Could you check a few things on this model? Use its own coordinates, in mm. Face numbers are marked on the shaded views. Give positions to 0.01 mm unless a question says otherwise; leave off trailing zeros. Order: outer loops, then holes, each group sorted by start corner. A loop starts at its lowest first (then second) coordinate and runs counter-clockwise, first axis right, second up. Notation, with made-up numbers: (21.5, -11.5) - (54.5, -11.5) arc R38 ccw to (54.5, 27.5) - close; hole circle Ø6 at (47.25, 46.5). An arc over 180 degrees is marked (long way). Put each result on its own line as item: value.
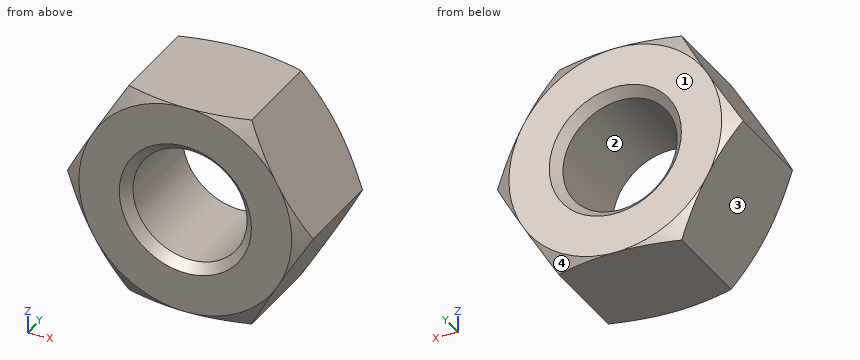
from build123d import *

# Parameters (mm, degrees)
BOSS_EXTRUDE1_DEPTH = 10
M12_TAPPED_HOLE1_D  = 10.2
CHAMFER1_SIZE       = 0.8


with BuildPart() as part:
    # Sketch1 → Boss-Extrude1 (new body)
    with BuildSketch(Plane(origin=(0, 0, 0), x_dir=(1, 0, 0), z_dir=(0, 1, 0))):
        Polygon((5.484827557, 9.5), (-5.484827557, 9.5), (-10.969655115, 0), (-5.484827557, -9.5), (5.484827557, -9.5), (10.969655115, 0), align=None)
    extrude(amount=BOSS_EXTRUDE1_DEPTH)

    # Sketch3 → Cut-Revolve1 (revolve, cut)
    with BuildSketch(Plane.XY):
        Polygon((9.5, 10), (10.969655115, 10), (10.969655115, 9.151494224), align=None)
        Polygon((10.969655115, 0.848505776), (9.5, 0), (10.969655115, 0), align=None)
    revolve(axis=Axis((0, 10, 0), (0, -1, 0)), mode=Mode.SUBTRACT)

    # M12 Tapped Hole1 (through all)
    with Locations(Plane(origin=(0, 10, 0), x_dir=(1, 0, 0), z_dir=(0, 1, 0))):
        with Locations((0, 0)):
            Hole(M12_TAPPED_HOLE1_D / 2)

    # Chamfer1
    chamfer1_edges = [part.edges().sort_by_distance(p)[0] for p in [
        (5.1, 10, 0),
        (5.1, 0, 0),
    ]]
    chamfer(chamfer1_edges, length=CHAMFER1_SIZE)


solid = part.part
1) Suppose I cut it at A-A, the plane y = 7.5. List the corners of the cut face in (x, z) for me.
Filled in:
outline: (-10.97, 0) - (-5.48, -9.5) - (5.48, -9.5) - (10.97, 0) - (5.48, 9.5) - (-5.48, 9.5) - close; hole circle Ø10.2 at (0, 0)
2) We'd pull the mould along X, two halves only. Please class the marked faces 1, 2, 3 and 4: pulls with the +X half, pulls with the -X half, needs draft (parallel to the pull), parting line crosses it, or undercut.
Filled in:
face 1: needs draft
face 2: undercut
face 3: pulls with the -X half
face 4: pulls with the +X half
3) Suppose I cut it at B-B, the plane y = 9.5. List the corners of the cut face in (x, z) for me, and give its area (3 significant figures).
Filled in:
outline: (-10.3, -1.16) - (-6.15, -8.34) arc R10.37 ccw to (-4.15, -9.5) - (4.15, -9.5) arc R10.37 ccw to (6.15, -8.34) - (10.3, -1.16) arc R10.37 ccw to (10.3, 1.16) - (6.15, 8.34) arc R10.37 ccw to (4.15, 9.5) - (-4.15, 9.5) arc R10.37 ccw to (-6.15, 8.34) - (-10.3, 1.16) arc R10.37 ccw to start; hole circle Ø10.8 at (0, 0)
area: 217 mm^2
4) If I drill on line 1 (Z direction, x = -3.75, y = 3.5); line 2 (X direction, y = 9.25, z = -3.5); line 3 (X direction, y = 5.75, z = -4), over which ranges is the centre line in solid material (lowest first)? Write a range as [from, to].
Filled in:
line 1: z = [-9.5, -3.46], [3.46, 9.5]
line 2: x = [-8.95, -3.78], [3.78, 8.95]
line 3: x = [-8.66, -3.16], [3.16, 8.66]
5) I'm going to push flat-ended pins straight in: pin 1 (5 mm diameter, centred on x = 8.5, y = 7.5, fed in from -Z); pin 2 (5 mm diameter, centred on x = 2.5, z = -1.5, fed in from +Y); pin 3 (6 mm diameter, centred on x = 0, z = 0, fed in from -Y); pin 4 (3 mm diameter, centred on y = 5.5, z = -2.5, fed in from -X). Where does each tip first touch, or does it pass through?
Filled in:
pin 1: stops at z = -8.61
pin 2: stops at y = 9.52
pin 3: passes through
pin 4: stops at x = -10.39
